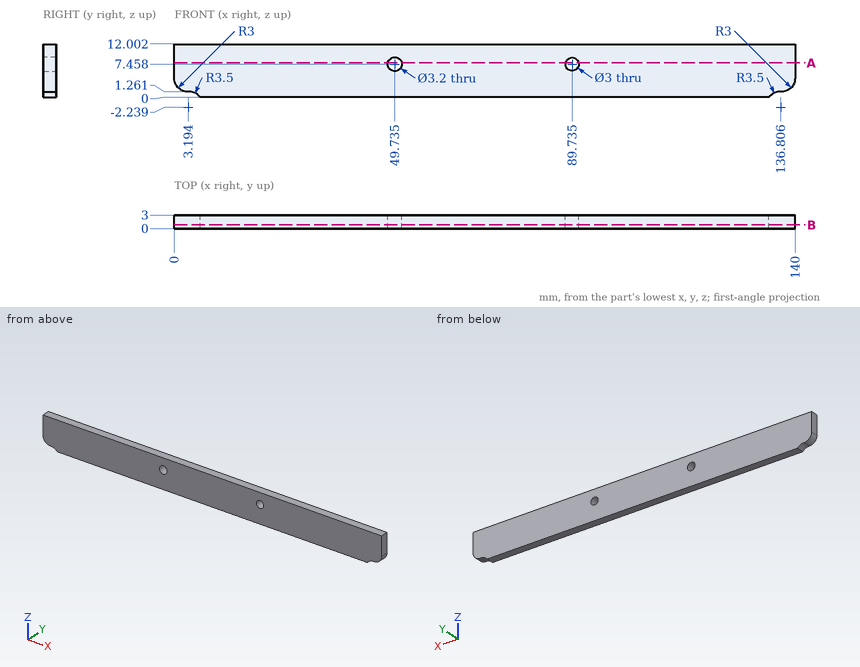
Geometry check sheet. Reference: drawing and pictorial views, mm from the part's lowest x, y, z. Coordinates: 2 decimals unless noted, no trailing zeros. Order: outer loops, then holes, each group sorted by start corner. A loop starts at its lowest first (then second) coordinate and runs counter-clockwise, first axis right, second up. Notation, with made-up numbers: M 5.25,-21 L 31.25,-21 A16 ccw 31.25,5 Z; hole C 57,-33 d3. An arc over 180 degrees is marked long. Return JSON: item names as keys, results as strings.
1) Gauge pin test, flat end, axial feed: pin 1 (2.5 mm diameter, centred on x = 89.74, z = 7.46, fed in from +Y) (3 decimals). Record the tip position at first contact, or that the pin passes through.
Answer list:
{"pin 1": "through"}
2) Cross-section at B-B, the plane y = 0.8. Count the separate pieces of the cut face and the enclosed holes in it, and give its area (3 significant figures).
Answer list:
{"separate pieces": "1", "enclosed holes": "2", "area": "1,650 mm2"}
3) Thickness scan on L1, parallel to X at y = 2.5, z = 8; L2, parallel to Z at x = 90, y = 0.95 (1 decimal); L3, parallel to X at y = 2.5, z = 7. Record the ranges inside material, lowest first. Write a range as [from, to].
Answer list:
{"L1": "[0, 48.23], [51.24, 88.34], [91.13, 140]", "L2": "[0, 6], [8.9, 12]", "L3": "[0, 48.2], [51.27, 88.31], [91.16, 140]"}
4) Cross-section at A-A, the plane z = 7.75. Record the boundary of the cut face in (x, y), and give its area (3 significant figures).
Answer list:
{"outline": "M 0,0 L 48.16,0 L 48.16,3 L 0,3 Z; M 51.31,0 L 88.26,0 L 88.26,3 L 51.31,3 Z; M 91.21,0 L 140,0 L 140,3 L 91.21,3 Z", "area": "402 mm2"}
